from build123d import *

# Parameters (mm, degrees)
F1_DEPTH = 25.4
F2_W     = 76.2
F2_H     = 9.652
F3_DEPTH = 25.4
F5_W     = 38.1
F5_H     = 66.802
F6_DEPTH = 25.4
F4_W     = 38.612633237
F4_H     = 47.752
F4_W_2   = 37.1750120858
F7_DEPTH = 25.4
F8_W     = 76.2
F8_H     = 76.2
F9_DEPTH = 25.4


with BuildPart() as f1:
    # F0 (on Front) → F1 (new body)
    with BuildSketch(Plane.XZ):
        Polygon((-58.6082313994, 110.9526419132), (-58.6082313994, -55.9253580868), (65.3437686006, -55.9253580868), (65.3437686006, 110.9526419132), (47.7265781481, 130.0026419132), (-38.1254218519, 130.0026419132), align=None)
    extrude(amount=F1_DEPTH)

    # F2 (on face) → F3 (cut)
    with BuildSketch(Plane.XZ.offset(25.4)):
        with Locations((3.3677686006, -41.4473580868)):
            Rectangle(F2_W, F2_H)
    extrude(amount=-F3_DEPTH, mode=Mode.SUBTRACT)

    # F5 (on face) → F6 (cut)
    with BuildSketch(Plane.XZ.offset(25.4)):
        with Locations((3.5901358351, -3.2203580868)):
            Rectangle(F5_W, F5_H)
    extrude(amount=-F6_DEPTH, mode=Mode.SUBTRACT)

    # F4 (on face) → F7 (cut)
    with BuildSketch(Plane.XZ.offset(25.4)):
        with Locations((-39.3019147809, -3.3473580868)):
            Rectangle(F4_W, F4_H)
        with Locations((46.7562625577, -3.3473580868)):
            Rectangle(F4_W_2, F4_H)
    extrude(amount=-F7_DEPTH, mode=Mode.SUBTRACT)

    # F8 (on face) → F9 (cut)
    with BuildSketch(Plane.XZ.offset(25.4)):
        with Locations((3.3754030544, 68.2806419132)):
            Rectangle(F8_W, F8_H)
    extrude(amount=-F9_DEPTH, mode=Mode.SUBTRACT)


solid = f1.part
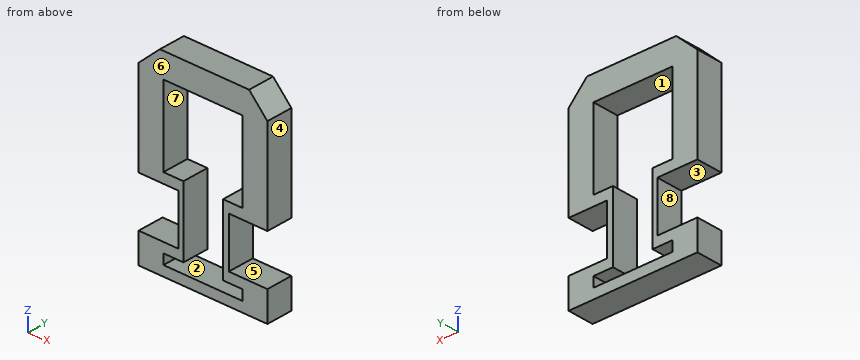
The listing builds one solid part. Answer for the finished solid, in the listing's coordinates (mm). Face numbers are marked on the shaded views. A direction names the side the tool comes from. Round coordinates to 2 decimals unless told otherwise and drop trailing zeros. Write each loop counter-clockwise with the first axis right and the second up, starting at its lowest first coordinate (ties: lowest second). Pieces come first, ordered by that corner, then holes. Notation, with made-up numbers: M 53.5,-7.75 L 100.5,-7.75 A20 cw 100.5,20.25 Z; hole C -12.5,33.25 d2. An arc over 180 degrees is marked long. Write each question's results on one line, items separated by ' | '. Start each with the question number.
Item 1: The mould has two halves that part along X. Classify the marked faces 1, 2, 3 and 4: +X half, -X half, draft (parallel to the pull), parting line (faces both ways), or undercut.
Item 2: Given pin 1 Ø1.5 at (x, z) = (22, -28) entering from -Y; pin 2 Ø12.5 at (y, z) = (-13, -7.5) entering from +X; pin 3 Ø12.5 at (x, y) = (-46, -7.5) entering from +Z; pin 4 Ø3 at (y, z) = (-3, -7) entering from -X, each flat-ended and moving along its own axis, determine where each tip first touches the part or whether it passes through.
Item 3: Which of the six approach directions +Z, -Z, +X, -X, +Y, -Y give full straight-line access (tool end or side, diameter ignored) to the marked faces 5, 6, 7 and 8?
Item 4: Find section C-C on x = 1. Write down the section's boundary in (y, z), and give its area (3 significant figures).
Item 5: Find section A-A on z = 39.5. Write down the section's boundary in (x, y), and give its area (3 significant figures).
Item 6: Straight lines are drawn through the part: probe 1 along Z at (x, y) = (-33, -2.25); probe 2 along X at (y, z) = (-20.25, -41.5); probe 3 along Z at (x, y) = (13, -3.25). For each, find the intervals that lie inside material, in ascending order.
Item 7: Find section D-D on x = -17.5. Write down the section's boundary in (y, z).
Item 8: Find section B-B on y = -11.75. Write down the section's boundary in (x, z).
Answer block:
1) face 1: undercut | face 2: undercut | face 3: draft | face 4: +X half
2) pin 1: stops at y = -25.4 | pin 2: stops at x = 28.17 | pin 3: stops at z = 128.49 | pin 4: stops at x = -20
3) face 5: +X, +Y, -Y | face 6: +Z, -Z, +X, -X, -Y | face 7: +Y, -Y | face 8: -X, +Y, -Y
4) outline: M -25.4,-55.93 L 0,-55.93 L 0,-46.27 L -25.4,-46.27 Z; M -25.4,106.38 L 0,106.38 L 0,130 L -25.4,130 Z | area: 845 mm²
5) outline: M -58.61,-25.4 L -34.72,-25.4 L -34.72,0 L -58.61,0 Z; M 41.48,-25.4 L 65.34,-25.4 L 65.34,0 L 41.48,0 Z | area: 1,210 mm²
6) probe 1: z = -55.93 to -46.27, -36.62 to -27.22, 20.53 to 30.18, 106.38 to 130 | probe 2: x = -58.61 to -34.73, 41.47 to 65.34 | probe 3: z = -55.93 to -46.27, 106.38 to 130
7) outline: M -25.4,-55.93 L 0,-55.93 L 0,-46.27 L -25.4,-46.27 Z; M -25.4,-36.62 L 0,-36.62 L 0,30.18 L -25.4,30.18 Z; M -25.4,106.38 L 0,106.38 L 0,130 L -25.4,130 Z
8) outline: M -58.61,-55.93 L 65.34,-55.93 L 65.34,-27.22 L 28.17,-27.22 L 28.17,20.53 L 65.34,20.53 L 65.34,110.95 L 47.73,130 L -38.13,130 L -58.61,110.95 L -58.61,20.53 L -20,20.53 L -20,-27.22 L -58.61,-27.22 Z; hole M -34.73,-46.27 L 41.47,-46.27 L 41.47,-36.62 L 22.64,-36.62 L 22.64,30.18 L 41.48,30.18 L 41.48,106.38 L -34.72,106.38 L -34.72,30.18 L -15.46,30.18 L -15.46,-36.62 L -34.73,-36.62 Z
